Geometry: final body of the model. Coordinates: model frame, mm. Coordinates: 2 decimals unless noted, no trailing zeros. Order: outer loops, then holes, each group sorted by start corner. A loop starts at its lowest first (then second) coordinate and runs counter-clockwise, first axis right, second up. Notation, with made-up numbers: M -29.5,41.25 L -16.5,41.25 A33 cw -16.5,70.25 Z; hole C -30.75,50.25 d11. An arc over 180 degrees is marked long. Use CSV: the item, a comma, the result in double quotes. Start each with the question number.
Q1. Section query B-B, the plane y = -17.25. Output: boundary loops of the cut face in (x, z).
Q2. Ray query, probe 1 along Z at (x, y) = (-12.5, -14.25); probe 2 along X at (y, z) = (-14.25, 23.5); probe 3 along Y at (x, z) = (-9, 27). Return the intervals inside material, ascending.
Q3. Section query A-A, the plane x = 18. Output: boundary loops of the cut face in (y, z), and give its area (3 significant figures).
Q4. First-contact query: P1, Ø5, axis at x = 17, y = -17, coming from the +Z side. Flat tip, straight axial feed; report the tip coordinate or a pass-through.
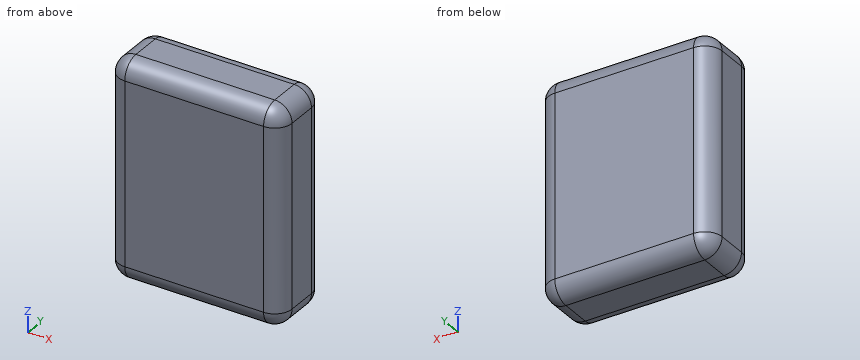
from build123d import *

# Parameters (mm, degrees)
F0_W     = 50.8
F0_H     = 63.5
F1_DEPTH = 19.05
F2_R     = 5.08
F3_R     = 5.08


with BuildPart() as f1:
    # F0 (on Front) → F1 (new body)
    with BuildSketch(Plane.XZ):
        Rectangle(F0_W, F0_H)
    extrude(amount=F1_DEPTH)

    # F2
    f2_edges = [f1.edges().sort_by_distance(p)[0] for p in [
        (-25.4, -19.05, 0),
        (0, -19.05, 31.75),
        (25.4, -19.05, 0),
        (0, -19.05, -31.75),
        (25.4, -9.525, -31.75),
        (-25.4, -9.525, -31.75),
        (25.4, -9.525, 31.75),
        (-25.4, -9.525, 31.75),
    ]]
    fillet(f2_edges, radius=F2_R)

    # F3
    f3_edges = [f1.edges().sort_by_distance(p)[0] for p in [
        (-25.4, 0, 0),
    ]]
    fillet(f3_edges, radius=F3_R)


solid = f1.part
Responses:
1,outline,"M -24.2,-26.67 A3.88 ccw -20.32,-30.55 L 20.32,-30.55 A3.88 ccw 24.2,-26.67 L 24.2,26.67 A3.88 ccw 20.32,30.55 L -20.32,30.55 A3.88 ccw -24.2,26.67 Z"
2,probe 1,"z = -31.74 to 31.74"
2,probe 2,"x = -25.39 to 25.39"
2,probe 3,"y = -19.04 to -0.01"
3,outline,"M -19.05,-26.67 A5.08 ccw -13.97,-31.75 L -5.08,-31.75 A5.08 ccw 0,-26.67 L 0,26.67 A5.08 ccw -5.08,31.75 L -13.97,31.75 A5.08 ccw -19.05,26.67 Z"
3,area,"1,190 mm²"
4,P1,"stops at z = 31.72"
